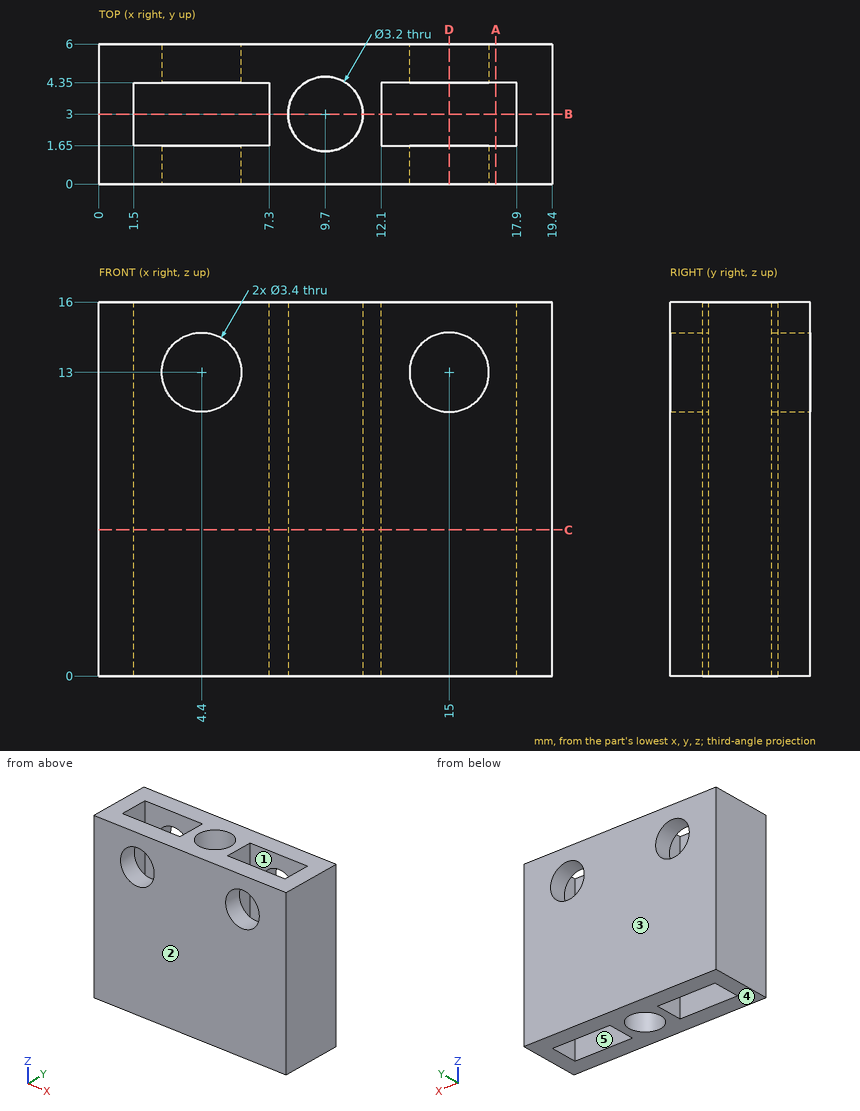
Geometry: see drawing. Coordinates: mm, zero at the bounding-box minimum. A direction names the side the tool comes from. Coordinates: 2 decimals unless noted, no trailing zeros. Loops run counter-clockwise (first coordinate to the right, second up) from the corner with the lowest first, then second, coordinate; pieces in that order, holes last. Notation, with made-up numbers: (56.5, 17.5) -> (97.5, 17.5) arc R18 ccw to (97.5, 27.5) -> close; hole circle Ø11 at (50.5, 32). An arc over 180 degrees is marked (long way). Write item = value, one per line. Start each with the question number.
Item 1: Reachability of the marked faces 1 and 2 from +Z, -Z, +X, -X, +Y, -Y: full face, straight path, thin tool, end or side. Return the list, or none.
Item 2: First-contact query: P1, Ø4.5, axis at x = 4.5, z = 5, coming from the -Y side. Flat tip, straight axial feed; report the tip coordinate or a pass-through.
Item 3: Cut plane C-C, the plane z = 6.25. Return loops of the section in (x, y), plus the area to 3 significant figures.
Item 4: Material intervals for line 1 (X direction, y = 3, z = 9); line 2 (Z direction, x = 4.4, y = 0.8); line 3 (Y direction, x = 17, z = 13.75), sorted ascending.
Item 5: Cut plane A-A, the plane x = 17. Return loops of the section in (y, z).
Item 6: Cut plane B-B, the plane y = 3. Return loops of the section in (x, z).
Item 7: Mould query, pull axis Y, two halves, no side actions, for the marked faces 3, 4 and 5. Classes: pulls with the +Y half, pulls with the -Y half, needs draft (parallel to the pull), parting line crosses it, or undercut.
Item 8: Cut plane D-D, the plane x = 15. Return loops of the section in (y, z).
Ans:
q1.face_1 = +Z, -Z
q1.face_2 = +Z, -Z, +X, -X, -Y
q2.P1 = 0
q3.outline = (0, 0) -> (19.4, 0) -> (19.4, 6) -> (0, 6) -> close; hole (1.5, 1.65) -> (7.3, 1.65) -> (7.3, 4.35) -> (1.5, 4.35) -> close; hole circle Ø3.2 at (9.7, 3); hole (12.1, 1.65) -> (17.9, 1.65) -> (17.9, 4.35) -> (12.1, 4.35) -> close
q3.area = 77.0 mm²
q4.line_1 = 0 to 1.5, 7.3 to 8.1, 11.3 to 12.1, 17.9 to 19.4
q4.line_2 = 0 to 11.3, 14.7 to 16
q4.line_3 = 0 to 1.65, 4.35 to 6
q5.outline = (0, 0) -> (1.65, 0) -> (1.65, 16) -> (0, 16) -> close; (4.35, 0) -> (6, 0) -> (6, 16) -> (4.35, 16) -> close
q6.outline = (0, 0) -> (1.5, 0) -> (1.5, 16) -> (0, 16) -> close; (7.3, 0) -> (8.1, 0) -> (8.1, 16) -> (7.3, 16) -> close; (11.3, 0) -> (12.1, 0) -> (12.1, 16) -> (11.3, 16) -> close; (17.9, 0) -> (19.4, 0) -> (19.4, 16) -> (17.9, 16) -> close
q7.face_3 = pulls with the +Y half
q7.face_4 = needs draft
q7.face_5 = undercut
q8.outline = (0, 0) -> (1.65, 0) -> (1.65, 11.3) -> (0, 11.3) -> close; (0, 14.7) -> (1.65, 14.7) -> (1.65, 16) -> (0, 16) -> close; (4.35, 0) -> (6, 0) -> (6, 11.3) -> (4.35, 11.3) -> close; (4.35, 14.7) -> (6, 14.7) -> (6, 16) -> (4.35, 16) -> close
